The listing builds one solid part. Answer for the finished solid, in the listing's coordinates (mm). A direction names the side the tool comes from. Round coordinates to 2 decimals unless told otherwise and drop trailing zeros. Write each loop counter-clockwise with the first axis right and the second up, starting at its lowest first coordinate (ties: lowest second). Pieces come first, ordered by that corner, then holes. Notation, with made-up numbers: (21.25, -9.75) - (43.25, -9.75) arc R34 cw to (43.25, 20.25) - close; hole circle Ø1 at (71.25, 52). An arc over 180 degrees is marked (long way). Answer in a Markdown table with one row per item.
from build123d import *

# Parameters (mm, degrees)
FILLET1_R             = 0.2
RECPAT_COUNT          = 2
RECPAT_ANGLE          = 90
CHAMFER_1_SIZE        = 0.5
CUT_EXTRUDE_START     = -1.932317225
CUT_EXTRUDE_1_DEPTH   = 0.992538955
CUT_EXTRUDE_1_2_DEPTH = 0.992538955
CUT_EXTRUDE_1_3_DEPTH = 0.992538955
CUT_EXTRUDE_1_4_DEPTH = 0.992538955


# Read off the part's stored shape, not the designer's step: Вытянуть1
with BuildPart() as part:
    # BodySke → Base-Revolve (revolve)
    with BuildSketch(Plane.XY, mode=Mode.PRIVATE) as base_revolve_sk:
        Polygon((3.05, 2), (3.05, 5), (2.05, 5), (2.05, 0), (23.05, 0), (23.05, 2), align=None)
    revolve(base_revolve_sk.sketch.rotate(Axis((-6.35, 0, 0), (1, 0, 0)), 90), axis=Axis((-6.35, 0, 0), (1, 0, 0)))

    # Fillet1
    fillet1_edges = [part.edges().sort_by_distance(p)[0] for p in [
        (3.05, 0, -2),
    ]]
    fillet(fillet1_edges, radius=FILLET1_R)

    # PanSke → Pan (revolve)
    with BuildSketch(Plane.XY):
        with BuildLine():
            Line((2.05, 4.424646879), (2.05, 0))
            Line((2.05, 0), (0, 0))
            ThreePointArc((0, 0), (0.537396082, 2.438237068), (2.05, 4.424646879))
        make_face()
    revolve(axis=Axis((0, 0, 0), (1, 0, 0)))

    # Sketch3 → Recess section 0
    with BuildSketch(Plane(origin=(0, 0, 0), x_dir=(0, 0, -1), z_dir=(1, 0, 0))):
        with BuildLine():
            Line((-0.515, 2.15), (0.515, 2.15))
            Line((0.515, 2.15), (0.515, -2.15))
            Line((0.515, -2.15), (-0.515, -2.15))
            Line((-0.515, -2.15), (-0.515, 2.15))
        make_face()
    # Sketch4 → Recess section 1
    with BuildSketch(Plane(origin=(2.34, 0, 0), x_dir=(0, 0, -1), z_dir=(1, 0, 0))):
        with BuildLine():
            Line((-0.37, 1.45), (0.37, 1.45))
            Line((0.37, 1.45), (0.37, -1.45))
            Line((0.37, -1.45), (-0.37, -1.45))
            Line((-0.37, -1.45), (-0.37, 1.45))
        make_face()
    recess = loft(mode=Mode.SUBTRACT)

    # RecPat: Recess ×2 about axis
    recpat_axis = Axis((0, 0, 0), (1, 0, 0))
    for i in range(1, RECPAT_COUNT):
        add(recess.rotate(recpat_axis, i * RECPAT_ANGLE / (RECPAT_COUNT - 1)), mode=Mode.SUBTRACT)

    # RecCorSke → RecessCore (revolve, cut)
    with BuildSketch(Plane.XY, mode=Mode.PRIVATE) as recesscore_sk:
        Polygon((0, 0), (0, 1.032809711), (2.6, 0.851), (2.876506661, 0), align=None)
    revolve(recesscore_sk.sketch.rotate(Axis((-3.175, 0, 0), (1, 0, 0)), 90), axis=Axis((-3.175, 0, 0), (1, 0, 0)), mode=Mode.SUBTRACT)

    # Фаска1
    chamfer_1_edges = [part.edges().sort_by_distance(p)[0] for p in [
        (23.05, 0, -2),
    ]]
    chamfer(chamfer_1_edges, length=CHAMFER_1_SIZE)

    # Вытянуть1 outline → Вытянуть1 (cut)
    with BuildSketch(Plane(origin=(0, 0, 0), x_dir=(0.9932989193126689, -0.08172287590474257, -0.08172287590474261), z_dir=(0.1155735994606204, 0.7023684015912574, 0.7023684015912578)).offset(CUT_EXTRUDE_START)):
        Polygon((-1, -0.919204654), (0.206895578, -0.216114133), (0.577867997, 0), (0.206895578, 0.216114133), (-1, 0.919204654), align=None)
    extrude(amount=CUT_EXTRUDE_1_DEPTH, mode=Mode.SUBTRACT)

    # Cut-Extrude 1 2 outline → Cut-Extrude 1 2 (cut)
    with BuildSketch(Plane(origin=(0, 0, 0), x_dir=(0.9932989193126689, -0.08172287590474257, 0.08172287590474261), z_dir=(0.1155735994606204, 0.7023684015912574, -0.7023684015912578)).offset(CUT_EXTRUDE_START)):
        Polygon((0.206895578, -0.216114133), (0.577867997, 0), (0.206895578, 0.216114133), (-1, 0.919204654), (-1, -0.919204654), align=None)
    extrude(amount=CUT_EXTRUDE_1_2_DEPTH, mode=Mode.SUBTRACT)

    # Cut-Extrude 1 3 outline → Cut-Extrude 1 3 (cut)
    with BuildSketch(Plane(origin=(0, 0, 0), x_dir=(0.9932989193126689, 0.08172287590474257, 0.08172287590474261), z_dir=(0.1155735994606204, -0.7023684015912574, -0.7023684015912578)).offset(CUT_EXTRUDE_START)):
        Polygon((0.206895578, -0.216114133), (0.577867997, 0), (0.206895578, 0.216114133), (-1, 0.919204654), (-1, -0.919204654), align=None)
    extrude(amount=CUT_EXTRUDE_1_3_DEPTH, mode=Mode.SUBTRACT)

    # Cut-Extrude 1 4 outline → Cut-Extrude 1 4 (cut)
    with BuildSketch(Plane(origin=(0, 0, 0), x_dir=(0.9932989193126689, 0.08172287590474257, -0.08172287590474261), z_dir=(0.1155735994606204, -0.7023684015912574, 0.7023684015912578)).offset(CUT_EXTRUDE_START)):
        Polygon((-1, -0.919204654), (0.206895578, -0.216114133), (0.577867997, 0), (0.206895578, 0.216114133), (-1, 0.919204654), align=None)
    extrude(amount=CUT_EXTRUDE_1_4_DEPTH, mode=Mode.SUBTRACT)


solid = part.part
(1) For faces 4 (the cylindrical face through (13, 2, 0)), 5 (the conical face through (1.6, -0.6, -0.7)), determine the directions among +Z, -Z, +X, -X, +Y, -Y from which every point of the face is accessible in a straight line to the end or side of a thin tool.
Checked values:
| item | result |
|---|---|
| face 4 | +X |
| face 5 | -X |
(2) Section A-A (z = 2.75) is taken. Give the vertices of the cut face in (x, y).
Checked values:
| item | result |
|---|---|
| outline | (2.05, -4.18) - (3.05, -4.18) - (3.05, 4.18) - (2.05, 4.18) - (2.05, 3.47) arc R5.11 ccw to (2.05, -3.47) - close |
(3) Flat-ended cylindrical pins translate along their axes: pin 1 (2 mm diameter, centred on x = 16.5, y = -2, fed in from +Z); pin 2 (5 mm diameter, centred on y = -3.5, z = -3.5, fed in from -X); pin 3 (4 mm diameter, centred on y = -0.5, z = 1, fed in from -X); pin 4 (0.5 mm diameter, centred on y = -1, z = 0, fed in from -X). Find the tip coordinate at first contact, or state that the pin passes through.
Checked values:
| item | result |
|---|---|
| pin 1 | stops at z = 1.73 |
| pin 2 | stops at x = 0.54 |
| pin 3 | stops at x = 0.09 |
| pin 4 | stops at x = 2.34 |
(4) Find the intervals of material crossed by line 1 (X direction, y = 4, z = -2.75); line 2 (Z direction, x = 15, y = 0.5); line 3 (Y direction, x = 2.25, z = -0.5), in increasing order.
Checked values:
| item | result |
|---|---|
| line 1 | x = 2.05 to 3.05 |
| line 2 | z = -1.94 to 1.94 |
| line 3 | y = -4.97 to -0.72, 0.72 to 4.97 |
(5) For a pull along Z with two mould halves and no side action, classify faces 1 (the flat face through (3.05, 1, -2.2)), 2 (the cylindrical face through (2.543, -0.22, -4.995)), 3 (the conical face through (2.863, -0.012, 0.039)) as pulls with the +Z half, pulls with the -Z half, needs draft (parallel to the pull), parting line crosses it, or undercut.
Checked values:
| item | result |
|---|---|
| face 1 | needs draft |
| face 2 | parting line crosses it |
| face 3 | undercut |
(6) Section C-C (y = -3) is taken. Give the vertices of the cut face in (x, z).
Checked values:
| item | result |
|---|---|
| outline | (2.05, -4) - (3.05, -4) - (3.05, 4) - (2.05, 4) - (2.05, 3.25) arc R4.96 ccw to (2.05, -3.25) - close |
(7) Section B-B (x = 19) is taken. Give the vertices of the cut face in (y, z).
Checked values:
| item | result |
|---|---|
| outline | circle Ø4 at (0, 0) |
